Can you work these out from the drawing? Everything is in mm from the part's minimum corner. Coordinates: 2 decimals unless noted, no trailing zeros. Loops run counter-clockwise (first coordinate to the right, second up) from the corner with the lowest first, then second, coordinate; pieces in that order, holes last. Notation, with made-up numbers: (75, 67.5) - (99, 67.5) arc R24 cw to (99, 90.5) - close; hole circle Ø4 at (57.25, -24). An arc over 180 degrees is marked (long way). Put each result on its own line as item: value. Start each with the question number.
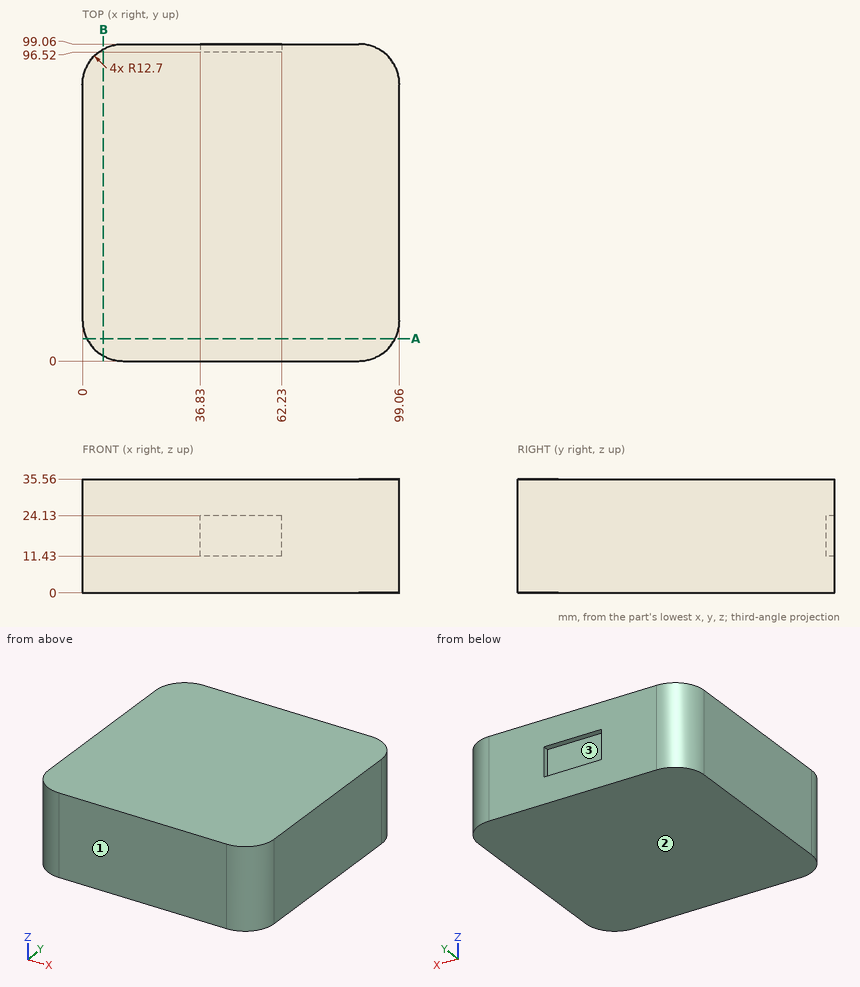
Q1. Please list where these lines run through material, in increasing order: line 1 along X through (y, z) = (86.5, 24.5); line 2 along Y through (x, z) = (40.5, 20.5); line 3 along Y through (x, z) = (87, 19). Write a range as [from, to].
Q2. I want a section at A-A on y = 7. List the corners of the cut face in (x, z) for me.
Q3. I want a section at B-B on x = 6.5. List the corners of the cut face in (y, z) for me.
Q4. We'd pull the mould along Z, two halves only. Please class the marked faces 1, 2 and 3: released by +Z, released by -Z, zero draft, split by the parting line, or undercut.
Q5. Will these pins go through, and if not, where does the flat tip stop? pin 1 (1.3 mm diameter, centred on y = 97.5, z = 15.5, fed in from -X); pin 2 (2 mm diameter, centred on y = 97.5, z = 15.5, fed in from +X).
Calculated:
1. line 1: [0, 99.06]
1. line 2: [0, 96.52]
1. line 3: [0.02, 99.04]
2. outline: (1.35, 0) - (97.71, 0) - (97.71, 35.56) - (1.35, 35.56) - close
3. outline: (1.62, 0) - (97.44, 0) - (97.44, 35.56) - (1.62, 35.56) - close
4. face 1: zero draft
4. face 2: released by -Z
4. face 3: undercut
5. pin 1: x = 5.54
5. pin 2: x = 94.01
